For this review, take the finished solid that the model builds, in its own axes (mm). Face numbers are marked on the shaded views. A direction names the side the tool comes from. Give positions to 0.01 mm unless a question says otherwise; leave off trailing zeros. Order: outer loops, then holes, each group sorted by start corner. A loop starts at its lowest first (then second) coordinate and runs counter-clockwise, first axis right, second up. Notation, with made-up numbers: M -21.75,87.25 L 34.25,87.25 A32 ccw 34.25,118.25 Z; hole C 30,14 d6. An arc over 180 degrees is marked long. Use CSV: the item, a comma, the result in double quotes. Start each with the question number.
(1) Wall thickness on L1, parallel to Y at x = 58, z = -1.95; L2, parallel to X at y = -0.25, z = -3.85; L3, parallel to Y at x = 30, z = -3.75: over which ranges is each line inside the solid? List them lowest first. Write a range as from..to.
(2) Tool access review of the marked faces 1 and 2: name each direction out of +Z, -Z, +X, -X, +Y, -Y from which nothing blocks a thin tool from reaching the whole face with its end or side.
(3) Draft analysis for pull direction Y (two halves, no side actions). For the marked faces 3 and 4, state which applies: pulls with the +Y half, pulls with the -Y half, needs draft (parallel to the pull), parting line crosses it, or undercut.
(4) Clearance check with flat-ended pins moving along their axes: P1, Ø3, axis at y = -5.5, z = -1.5, coming from the +X side; P2, Ø3, axis at y = 7.5, z = -2.5, coming from the +X side; P3, Ø6, axis at x = 5.5, y = 1.5, coming from the +Z side. State where each tip first meets the part, or that it passes through.
(5) Consider section B-B (x = 149). Write out the cut boundary in (y, z).
(6) Consider section A-A (z = -1.2). Give the number of separate pieces and of enclosed holes in the cut face, and give its area (3 significant figures).
```python
from build123d import *

# Parameters (mm, degrees)
EXTRUDE_1_DEPTH      = 5
SKETCH_1_3_R         = 1.1
CUT_EXTRUDE_2_DEPTH  = 187.33571853
SKETCH_1_4_R         = 2.55
CUT_EXTRUDE_3_DEPTH  = 2.6
SKETCH_2_R           = 1.25
CUT_EXTRUDE_4_DEPTH  = 187.33571853
CUT_EXTRUDE_START    = -5
SKETCH_2_3_R         = 2
CUT_EXTRUDE_5_DEPTH  = 2.5
SKETCH_3_W           = 59
SKETCH_3_H           = 2.6
CUT_EXTRUDE_6_DEPTH  = 188.138985783
CUT_EXTRUDE_7_DEPTH  = 187.33571853
SKETCH_5_W           = 210.843247287
SKETCH_5_H           = 25.236064347
CUT_EXTRUDE_8_DEPTH  = 187.33571853
SKETCH_6_R           = 13.5
CUT_EXTRUDE_9_DEPTH  = 3
SKETCH_7_R           = 4.5
CUT_EXTRUDE_10_DEPTH = 187.33571853
SKETCH_8_R           = 1.6
SKETCH_8_R_2         = 0.9
CUT_EXTRUDE_11_DEPTH = 187.33571853


with BuildPart() as part:
    # 草图1 → 凸台-拉伸1 (new body)
    with BuildSketch(Plane.XY):
        with BuildLine():
            Line((0, -10), (176, -10))
            ThreePointArc((176, -10), (186, 0), (176, 10))
            Line((176, 10), (0, 10))
            ThreePointArc((0, 10), (-10, 0), (0, -10))
        make_face()
    extrude(amount=EXTRUDE_1_DEPTH)

    # 草图1<3> → 切除-拉伸2 (cut, through all)
    with BuildSketch(Plane.XY):
        with Locations((88, 0)):
            Circle(SKETCH_1_3_R)
        Circle(SKETCH_1_3_R)
    extrude(amount=CUT_EXTRUDE_2_DEPTH, mode=Mode.SUBTRACT)

    # 草图1<4> → 切除-拉伸3 (cut)
    with BuildSketch(Plane.XY):
        with Locations((88, 0)):
            Circle(SKETCH_1_4_R)
        Circle(SKETCH_1_4_R)
    extrude(amount=CUT_EXTRUDE_3_DEPTH, mode=Mode.SUBTRACT)

    # 草图2 → 切除-拉伸4 (cut, through all)
    with BuildSketch(Plane(origin=(0, 0, 0), x_dir=(-1, 0, 0), z_dir=(0, 0, -1))):
        with Locations((-121, -6)):
            Circle(SKETCH_2_R)
        with Locations((-121, 6)):
            Circle(SKETCH_2_R)
        with Locations((-114, 0)):
            Circle(SKETCH_2_R)
        with Locations((-58, 7)):
            Circle(SKETCH_2_R)
        with Locations((-30, 7)):
            Circle(SKETCH_2_R)
        with Locations((-58, -7)):
            Circle(SKETCH_2_R)
        with Locations((-30, -7)):
            Circle(SKETCH_2_R)
    extrude(amount=-CUT_EXTRUDE_4_DEPTH, mode=Mode.SUBTRACT)

    # 草图2<3> → 切除-拉伸5 (cut)
    with BuildSketch(Plane(origin=(0, 0, 0), x_dir=(-1, 0, 0), z_dir=(0, 0, -1)).offset(CUT_EXTRUDE_START)):
        with Locations(Location((-121, -6, 0), (0, 0, 180))):
            Circle(SKETCH_2_3_R)
        with Locations(Location((-121, 6, 0), (0, 0, 180))):
            Circle(SKETCH_2_3_R)
        with Locations(Location((-114, 0, 0), (0, 0, 180))):
            Circle(SKETCH_2_3_R)
        with Locations(Location((-58, 7, 0), (0, 0, 180))):
            Circle(SKETCH_2_3_R)
        with Locations(Location((-30, 7, 0), (0, 0, 180))):
            Circle(SKETCH_2_3_R)
        with Locations(Location((-58, -7, 0), (0, 0, 180))):
            Circle(SKETCH_2_3_R)
        with Locations(Location((-30, -7, 0), (0, 0, 180))):
            Circle(SKETCH_2_3_R)
    extrude(amount=CUT_EXTRUDE_5_DEPTH, mode=Mode.SUBTRACT)

    # 草图3 → 切除-拉伸6 (cut, through all)
    with BuildSketch(Plane(origin=(0, 10, 0), x_dir=(1, 0, 0), z_dir=(0, 1, 0))):
        with Locations((156.5, -1.3)):
            Rectangle(SKETCH_3_W, SKETCH_3_H)
    extrude(amount=-CUT_EXTRUDE_6_DEPTH, mode=Mode.SUBTRACT)

    # 草图4 → 切除-拉伸7 (cut, through all)
    with BuildSketch(Plane.XY.offset(5)):
        with BuildLine():
            Line((164.2, -2.4), (154, -2.4))
            ThreePointArc((154, -2.4), (152.4, -4), (154, -5.6))
            Line((154, -5.6), (164.2, -5.6))
            ThreePointArc((164.2, -5.6), (165.8, -4), (164.2, -2.4))
        make_face()
        with BuildLine():
            ThreePointArc((154, 5.6), (152.4, 4), (154, 2.4))
            Line((154, 2.4), (164.2, 2.4))
            ThreePointArc((164.2, 2.4), (165.8, 4), (164.2, 5.6))
            Line((164.2, 5.6), (154, 5.6))
        make_face()
    extrude(amount=-CUT_EXTRUDE_7_DEPTH, mode=Mode.SUBTRACT)

    # 镜向1: part across plane


with BuildPart() as part_1:
    add(part.part)
    add(part.part.mirror(Plane.XY))

    # 草图5 → 切除-拉伸8 (cut, through all)
    with BuildSketch(Plane.XY):
        with Locations((85.761316873, -1.017583239)):
            Rectangle(SKETCH_5_W, SKETCH_5_H)
    extrude(amount=CUT_EXTRUDE_8_DEPTH, mode=Mode.SUBTRACT)

    # 草图6 → 切除-拉伸9 (cut)
    with BuildSketch(Plane.XY):
        Circle(SKETCH_6_R)
    extrude(amount=-CUT_EXTRUDE_9_DEPTH, mode=Mode.SUBTRACT)

    # 草图7 → 切除-拉伸10 (cut, through all)
    with BuildSketch(Plane(origin=(0, 0, -5), x_dir=(-1, 0, 0), z_dir=(0, 0, -1))):
        Circle(SKETCH_7_R)
    extrude(amount=-CUT_EXTRUDE_10_DEPTH, mode=Mode.SUBTRACT)

    # 草图8 → 切除-拉伸11 (cut, through all)
    with BuildSketch(Plane(origin=(0, 0, -5), x_dir=(-1, 0, 0), z_dir=(0, 0, -1))):
        with Locations((-11.5, 0)):
            Circle(SKETCH_8_R)
        with Locations((-8, 7)):
            Circle(SKETCH_8_R_2)
        with Locations((-8, -7)):
            Circle(SKETCH_8_R_2)
        with Locations((-20.5, 0)):
            Circle(SKETCH_8_R_2)
    extrude(amount=-CUT_EXTRUDE_11_DEPTH, mode=Mode.SUBTRACT)


solid = part_1.part
```
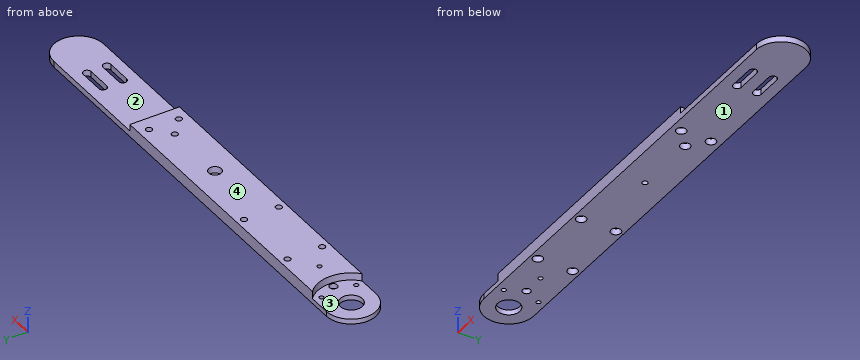
Check result:
1,L1,"y = -10..-8.25, -5.75..5.75, 8.25..10"
1,L2,"x = -10..-4.49, 4.49..9.92, 13.08..19.64, 21.36..86.93, 89.07..112.02, 115.98..186"
1,L3,"y = -10..-9, -5..5, 9..10"
2,face 1,"-Z, +X, -X, +Y, -Y"
2,face 2,"+Z, +X, +Y, -Y"
3,face 3,"undercut"
3,face 4,"needs draft"
4,P1,"stops at x = 184.94"
4,P2,"stops at x = 184"
4,P3,"stops at z = -3"
5,outline,"M -10,-5 L 10,-5 L 10,-2.6 L -10,-2.6 Z"
6,separate pieces,"1"
6,enclosed holes,"9"
6,area,"2,240 mm^2"
